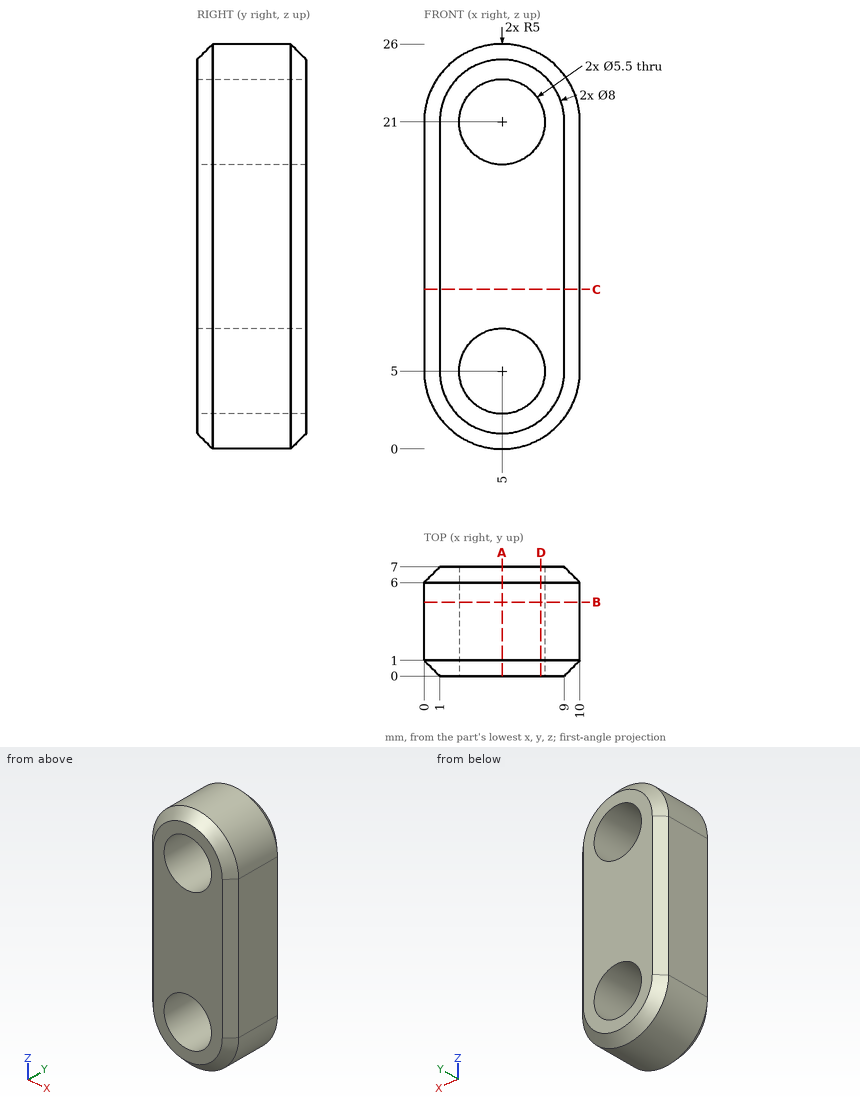
For this review, use the dimensioned drawing (mm, ordinates from the lowest corner) and the shaded views. Coordinates: 2 decimals unless noted, no trailing zeros. Loops run counter-clockwise (first coordinate to the right, second up) from the corner with the lowest first, then second, coordinate; pieces in that order, holes last.
1. Add section B-B, the plane y = 4.75. Give the boundary of the cut face in (x, z), then the cut area to 3 significant figures.
2. For line 1 (Z direction, x = 3, y = 6.75); line 2 (X direction, y = 5.5, z = 21); line 3 (Z direction, x = 6.5, y = 4), list the stretches that pass through material, from the lowest coordinate up.
3. Add section A-A, the plane x = 5. Give the boundary of the cut face in (y, z), then the cut area to 3 significant figures.
4. Add section D-D, the plane x = 7.5. Count the separate pieces of the cut face and the enclosed holes in it, then the cut area to 3 significant figures.
5. Add section C-C, the plane z = 10.25. Give the boundary of the cut face in (x, y).
Result:
1. outline: (0, 5) arc R5 ccw to (10, 5) - (10, 21) arc R5 ccw to (0, 21) - close; hole circle Ø5.5 at (5, 5); hole circle Ø5.5 at (5, 21)
1. area: 191 mm2
2. line 1: z = 1.25 to 3.11, 6.89 to 19.11, 22.89 to 24.75
2. line 2: x = 0 to 2.25, 7.75 to 10
2. line 3: z = 0.23 to 2.7, 7.3 to 18.7, 23.3 to 25.77
3. outline: (0, 1) - (1, 0) - (6, 0) - (7, 1) - (7, 2.25) - (0, 2.25) - close; (0, 7.75) - (7, 7.75) - (7, 18.25) - (0, 18.25) - close; (0, 23.75) - (7, 23.75) - (7, 25) - (6, 26) - (1, 26) - (0, 25) - close
3. area: 103 mm2
4. separate pieces: 3
4. enclosed holes: 0
4. area: 138 mm2
5. outline: (0, 1) - (1, 0) - (9, 0) - (10, 1) - (10, 6) - (9, 7) - (1, 7) - (0, 6) - close
